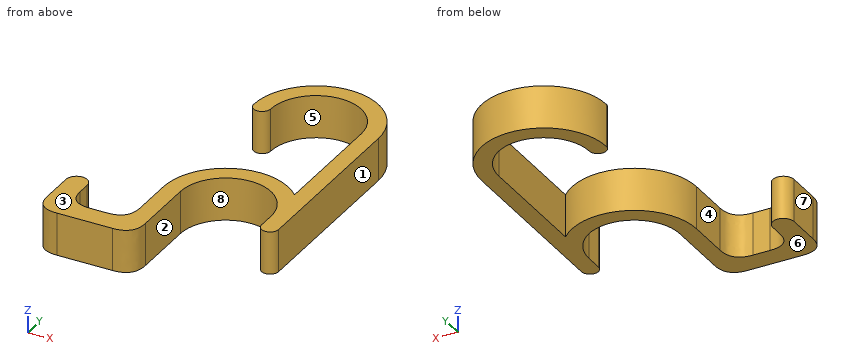
from build123d import *

# Parameters (mm, degrees)
F1_DEPTH    = 10
F2_T1_DEPTH = 10
F2_T3_DEPTH = 35


# Not quite as in the source:
# - a fillet or chamfer that OpenCascade refuses, or shapes differently, is made with other operations: its cross-section is extruded or revolved along the edge and cut away or added


with BuildPart() as f1:
    # F0 (on Top) → F1 (new body)
    with BuildSketch(Plane.XY):
        with BuildLine():
            Line((14.6, -4), (14.6, 38.55))
            ThreePointArc((14.6, 38.55), (0, 53.15), (-14.6, 38.55))
            ThreePointArc((-14.6, 38.55), (-12.6, 36.55), (-10.6, 38.55))
            ThreePointArc((-10.6, 38.55), (0, 49.15), (10.6, 38.55))
            Line((10.6, 38.55), (10.6, 10.0399203184))
            ThreePointArc((10.6, 10.0399203184), (-5.4037024344, 13.5631854665), (-14.6, 0))
            Line((-14.6, 0), (-14.6, -15))
            Line((-14.6, -15), (-28.6, -15))
            Line((-28.6, -15), (-28.6, -7))
            ThreePointArc((-28.6, -7), (-31.1, -4.5), (-33.6, -7))
            Line((-33.6, -7), (-33.6, -20))
            Line((-33.6, -20), (-10.6, -20))
            Line((-10.6, -20), (-10.6, 0))
            ThreePointArc((-10.6, 0), (0, 10.6), (10.6, 0))
            Line((10.6, 0), (10.6, -4))
            ThreePointArc((10.6, -4), (12.6, -6), (14.6, -4))
        make_face()
    extrude(amount=F1_DEPTH)

    # F2: fillet of radius 5 on 4 edges, made by hand

    # F2_s2 → F2_t1 (join)
    with BuildSketch(Plane.XY):
        with BuildLine():
            add(Edge.make_bspline(
                [(-14.6, -10), (-14.6, -15), (-19.6, -15)],
                knots=[0, 0, 0, 1, 1, 1], degree=2, weights=[1, 1, 1]))
            Line((-19.6, -15), (-14.6, -15))
            Line((-14.6, -15), (-14.6, -10))
        make_face()
        with BuildLine():
            add(Edge.make_bspline(
                [(-23.6, -15), (-28.6, -15), (-28.6, -10)],
                knots=[0, 0, 0, 1, 1, 1], degree=2, weights=[1, 1, 1]))
            Line((-28.6, -10), (-28.6, -15))
            Line((-28.6, -15), (-23.6, -15))
        make_face()
    extrude(amount=F2_T1_DEPTH)

    # F2_s4 → F2_t3 (cut)
    with BuildSketch(Plane.XY.offset(-12.5)):
        with BuildLine():
            add(Edge.make_bspline(
                [(-33.6, -15), (-33.6, -20), (-28.6, -20)],
                knots=[0, 0, 0, 1, 1, 1], degree=2, weights=[1, 1, 1]))
            Line((-28.6, -20), (-33.6, -20))
            Line((-33.6, -20), (-33.6, -15))
        make_face()
        with BuildLine():
            add(Edge.make_bspline(
                [(-10.6, -15), (-10.6, -20), (-15.6, -20)],
                knots=[0, 0, 0, 1, 1, 1], degree=2, weights=[1, 1, 1]))
            Line((-15.6, -20), (-10.6, -20))
            Line((-10.6, -20), (-10.6, -15))
        make_face()
    extrude(amount=F2_T3_DEPTH, mode=Mode.SUBTRACT)


solid = f1.part
Check sheet for the modelled part. Datum: model origin and axes. Units: mm. Face numbers are marked on the shaded views. A direction names the side the tool comes from. Give positions to 0.01 mm unless a question says otherwise; leave off trailing zeros. Loops run counter-clockwise (first coordinate to the right, second up) from the corner with the lowest first, then second, coordinate; pieces in that order, holes last. Notation, with made-up numbers: M -35.5,19 L 14.5,19 A24 cw 14.5,44 Z; hole C 54,-28 d9. An arc over 180 degrees is marked long. Return JSON: item names as keys, results as strings. Group by question number.
1. Go/stop test with flat-tipped pins: pin 1 (1 mm diameter, centred on x = 8.5, y = 33, fed in from -Z); pin 2 (2 mm diameter, centred on y = 26.5, z = 3, fed in from -X); pin 3 (2 mm diameter, centred on x = -22, z = 3.5, fed in from +Y); pin 4 (1.2 mm diameter, centred on y = -2, z = 4.5, fed in from -X). Record where each tip stops, or that it passes through.
2. Mould release check, pull along X, two halves, no side actions. Record for the marked faces 6, 7 and 8: released by +X, released by -X, zero draft, split by the parting line, or undercut.
3. Cross-section at D-D on x = 12.6. Record the boundary of the cut face in (y, z), plus the area to 3 significant figures.
4. Tool access check on the marked faces 1, 2, 3, 4 and 5. Record the directions out of +Z, -Z, +X, -X, +Y, -Y that give a thin tool (end or side, any length) a straight path to the whole face; none if there is none.
5. Cross-section at B-B on x = -6. Record the boundary of the cut face in (y, z).
6. Cross-section at C-C on y = 16.5. Record the boundary of the cut face in (x, z), plus the area to 3 significant figures.
7. Thickness scan on L1, parallel to X at y = -3.5, z = 4.25; L2, parallel to X at y = -5.5, z = 4.5; L3, parallel to X at y = -8.5, z = 4. Record the ranges inside material, lowest first.
8. Cross-section at A-A on y = 43. Record the boundary of the cut face in (x, z), plus the area to 3 significant figures.
Return value:
{
 "1": {"pin 1": "through", "pin 2": "x = 10.6", "pin 3": "y = -15", "pin 4": "x = -14.6"},
 "2": {"face 6": "zero draft", "face 7": "released by -X", "face 8": "undercut"},
 "3": {"outline": "M -6,0 L 45.93,0 L 45.93,10 L -6,10 Z", "area": "519 mm^2"},
 "4": {"face 1": "+Z, -Z, +X, +Y, -Y", "face 2": "+Z, -Z, -Y", "face 3": "+Z, +X, -X, +Y, -Y", "face 4": "+Z, -Z, +Y", "face 5": "+Z, -Z"},
 "5": {"outline": "M 8.74,0 L 13.31,0 L 13.31,10 L 8.74,10 Z; M 47.29,0 L 51.86,0 L 51.86,10 L 47.29,10 Z"},
 "6": {"outline": "M 10.6,0 L 14.6,0 L 14.6,10 L 10.6,10 Z", "area": "40.0 mm^2"},
 "7": {"L1": "-14.6 to -10.6, 10.6 to 14.6", "L2": "-33.1 to -29.1, -14.6 to -10.6, 11.28 to 13.92", "L3": "-33.6 to -28.6, -14.6 to -10.6"},
 "8": {"outline": "M -13.91,0 L -9.62,0 L -9.62,10 L -13.91,10 Z; M 9.62,0 L 13.91,0 L 13.91,10 L 9.62,10 Z", "area": "85.7 mm^2"}
}
